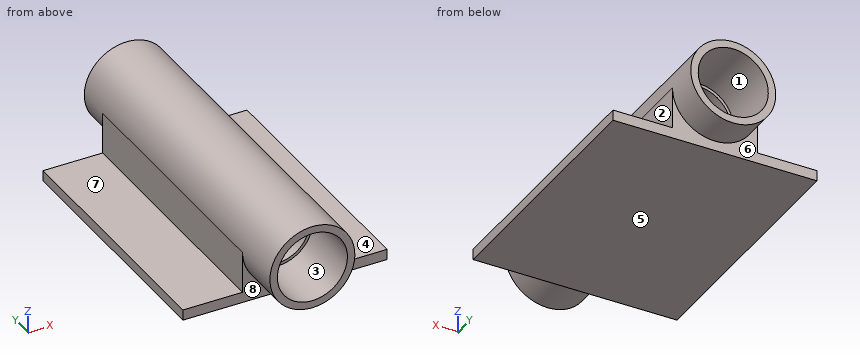
from build123d import *

# Parameters (mm, degrees)
BOSS_EXTRUDE1_START = -153.2
BOSS_EXTRUDE1_DEPTH = 153.2


with BuildPart() as part:
    # Sketch12 → Revolve1 (revolve)
    with BuildSketch(Plane.XY, mode=Mode.PRIVATE) as revolve1_sk:
        Polygon((-25.399999994, 0), (-25.399999994, 203.2), (-20.955, 203.2), (-20.955, 165.1), (-19.177, 165.1), (-19.177, 38.1), (-20.955, 38.1), (-20.955, 0), align=None)
    revolve(revolve1_sk.sketch.rotate(Axis((0, 0, 0), (0, 1, 0)), 270), axis=Axis((0, 0, 0), (0, 1, 0)))

    # Sketch13 → Boss-Extrude1 (add)
    with BuildSketch(Plane(origin=(0, 30, 0), x_dir=(-1, 0, 0), z_dir=(0, -1, 0)).offset(BOSS_EXTRUDE1_START)):
        with BuildLine():
            Line((61, 24.899999994), (61, 31.249999994))
            Line((61, 31.249999994), (-61, 31.249999994))
            Line((-61, 31.249999994), (-61, 24.899999994))
            Line((-61, 24.899999994), (-25.399999994, 24.899999994))
            Line((-25.399999994, 24.899999994), (-25.399999994, 0))
            ThreePointArc((-25.399999994, 0), (0, 25.399999994), (25.399999994, 0))
            Line((25.399999994, 0), (25.399999994, 24.899999994))
            Line((25.399999994, 24.899999994), (61, 24.899999994))
        make_face()
    extrude(amount=BOSS_EXTRUDE1_DEPTH)


solid = part.part
Can you work these out from the model? Positions are in its coordinate system, mm. Face numbers are marked on the shaded views. A direction names the side the tool comes from. Coordinates: 2 decimals unless noted, no trailing zeros. Order: outer loops, then holes, each group sorted by start corner. A loop starts at its lowest first (then second) coordinate and runs counter-clockwise, first axis right, second up. Notation, with made-up numbers: M -25.5,19 L -15.5,19 A19 ccw -15.5,25 Z; hole C -10.5,66 d9. An arc over 180 degrees is marked long. Answer as CSV lines item,"result".
(1) I'm going to push flat-ended pins straight in: pin 1 (6 mm diameter, centred on x = 32.5, z = -22.5, fed in from +Y); pin 2 (9.5 mm diameter, centred on x = -15.5, z = -12.5, fed in from +Y); pin 3 (3 mm diameter, centred on x = -22.5, y = 164.5, fed in from +Z); pin 4 (10.5 mm diameter, centred on x = 35.5, y = 137, fed in from +Z). Where does each tip first touch, or does it pass through?
Geometry check:
pin 1,"y = 183.2"
pin 2,"y = 203.2"
pin 3,"z = 14.29"
pin 4,"z = -24.9"
(2) On a 3-axis mill with a long thin cutter (end or side, diameter ignored), from which of +Z, -Z, +X, -X, +Y, -Y can I reach the whole of each face in a straight line? I mean the marked faces 5, 6, 7 and 8. Say none if no direction works.
Geometry check:
face 5,"-Z, +X, -X, +Y, -Y"
face 6,"-Z, +Y"
face 7,"+Z, -X, +Y, -Y"
face 8,"-Z, -Y"
(3) If we mould it in two halves opening along Z, with no side actions, what happens to the marked faces 1, 2, 3 and 4? For each: released by +Z, released by -Z, zero draft, split by the parting line, or undercut.
Geometry check:
face 1,"undercut"
face 2,"zero draft"
face 3,"undercut"
face 4,"released by +Z"
(4) Suppose I cut it at D-D on y = 175. Please give me the cut outline in (x, z) (3 decimals).
Geometry check:
outline,"M -61,-31.25 L 61,-31.25 L 61,-24.9 L 25.4,-24.9 L 25.4,0 A25.4 ccw -25.4,0 L -25.4,-24.9 L -61,-24.9 Z; hole C 0,0 d41.91"
(5) Suppose I cut it at A-A on x = 0. Please give me the cut outline in (y, z) (3 decimals), plus the area to 3 significant figures.
Geometry check:
outline,"M 0,-25.4 L 30,-25.4 L 30,-31.25 L 183.2,-31.25 L 183.2,-25.4 L 203.2,-25.4 L 203.2,-20.955 L 165.1,-20.955 L 165.1,-19.177 L 38.1,-19.177 L 38.1,-20.955 L 0,-20.955 Z; M 0,20.955 L 38.1,20.955 L 38.1,19.177 L 165.1,19.177 L 165.1,20.955 L 203.2,20.955 L 203.2,25.4 L 0,25.4 Z"
area,"3,150 mm^2"
(6) Please list where these lines run through material, in increasing order: L1, parallel to X at y = 183, z = 0 (3 decimals); L2, parallel to X at y = 86, z = 0; L3, parallel to Z at x = 7.5, y = 13.
Geometry check:
L1,"-25.4 to -20.955, 20.955 to 25.4"
L2,"-25.4 to -19.18, 19.18 to 25.4"
L3,"-24.27 to -19.57, 19.57 to 24.27"
(7) Suppose I cut it at B-B on y = 55. Please give me the cut outline in (x, z).
Geometry check:
outline,"M -61,-31.25 L 61,-31.25 L 61,-24.9 L 25.4,-24.9 L 25.4,0 A25.4 ccw -25.4,0 L -25.4,-24.9 L -61,-24.9 Z; hole C 0,0 d38.35"
(8) Suppose I cut it at C-C on z = -8.5. Please give me the cut outline in (x, y).
Geometry check:
outline,"M -25.4,30 L -23.94,30 L -23.94,0 L -19.15,0 L -19.15,38.1 L -17.19,38.1 L -17.19,165.1 L -19.15,165.1 L -19.15,203.2 L -23.94,203.2 L -23.94,183.2 L -25.4,183.2 Z; M 17.19,38.1 L 19.15,38.1 L 19.15,0 L 23.94,0 L 23.94,30 L 25.4,30 L 25.4,183.2 L 23.94,183.2 L 23.94,203.2 L 19.15,203.2 L 19.15,165.1 L 17.19,165.1 Z"
